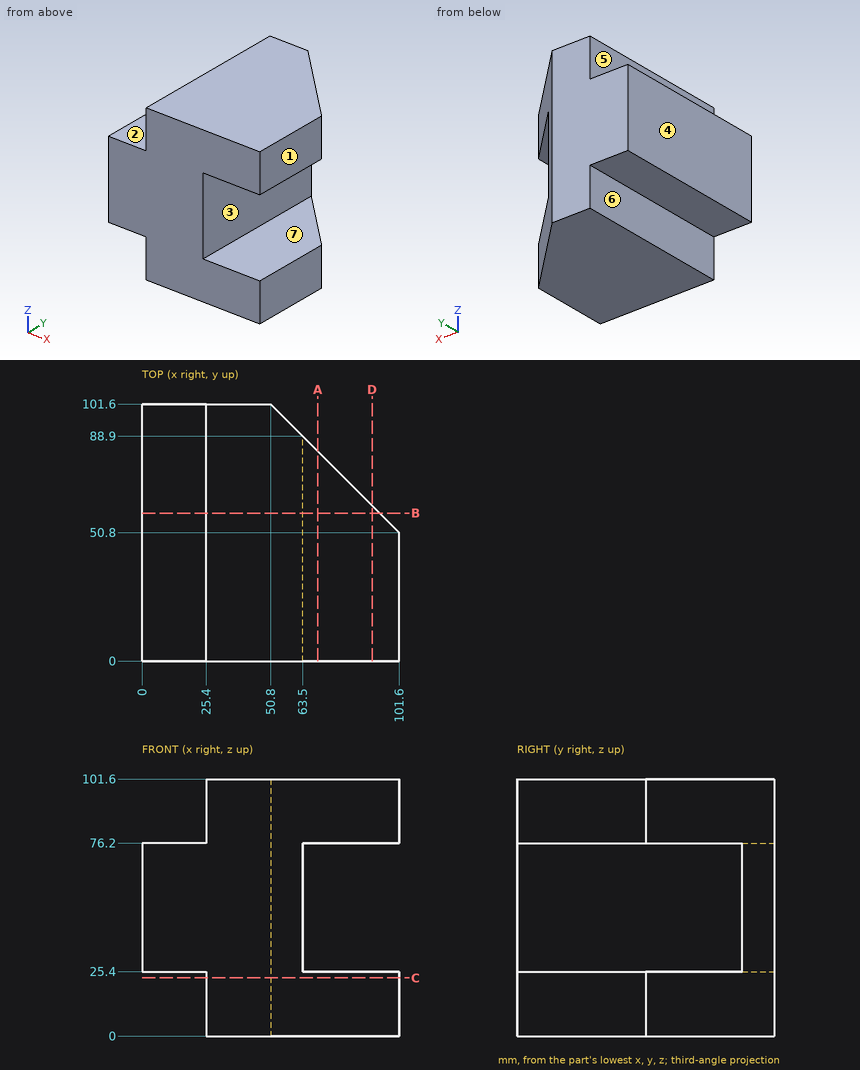
Part print with two shaded views. Sizes in mm from the minimum x, y, z corner. A direction names the side the tool comes from. Round coordinates to 2 decimals unless told otherwise and drop trailing zeros. Order: outer loops, then holes, each group sorted by start corner. A loop starts at its lowest first (then second) coordinate and runs counter-clockwise, first axis right, second up. Notation, with made-up numbers: M 13,66.5 L 24,66.5 A19 ccw 24,88.5 Z; hole C -3.75,-24.75 d7. An arc over 180 degrees is marked long. Use CSV: the item, a comma, the result in double quotes. Start each with the question number.
(1) Cut at B-B on y = 58.5. List the corners of the cut face in (x, z), then the cut area to 3 significant figures.
(2) Cut at D-D on x = 91. List the corners of the cut face in (y, z).
(3) Flat gauge pins, fed straight in: P1, Ø2, axis at x = 65, z = 67, coming from the -Y side (1 decimal); P2, Ø12.5, axis at x = 12, y = 64.5, coming from the +Z side; P3, Ø1, axis at y = 66.5, z = 79.5, coming from the +X side; P4, Ø15, axis at y = 36.5, z = 50, coming from the +X side. Where does each tip first touch, or does it go through?
(4) Cut at A-A on x = 69.5. List the corners of the cut face in (y, z), then the cut area to 3 significant figures.
(5) Mould opens along Z. For the marked faces 1, 2 and 3 say: +Z half, -Z half, draft (parallel to the pull), parting line (faces both ways), or undercut.
(6) Tool access for the marked faces 4, 5, 6 and 7: list every direction of +Z, -Z, +X, -X, +Y, -Y with a clear straight run to the whole face (end or side of a thin tool).
(7) Drill centre lines: probe 1 along Z at (x, y) = (96, 26); probe 2 along X at (y, z) = (61, 44.5); probe 3 along X at (y, z) = (25, 79). Where is each one in solid material? Low to high.
(8) Cut at C-C on z = 23. List the corners of the cut face in (x, y), then the cut area to 3 significant figures.
Findings:
1,outline,"M 0,25.4 L 25.4,25.4 L 25.4,0 L 93.9,0 L 93.9,25.4 L 63.5,25.4 L 63.5,76.2 L 93.9,76.2 L 93.9,101.6 L 25.4,101.6 L 25.4,76.2 L 0,76.2 Z"
1,area,"6,710 mm^2"
2,outline,"M 0,0 L 61.4,0 L 61.4,25.4 L 0,25.4 Z; M 0,76.2 L 61.4,76.2 L 61.4,101.6 L 0,101.6 Z"
3,P1,"passes through"
3,P2,"stops at z = 76.2"
3,P3,"stops at x = 86.4"
3,P4,"stops at x = 63.5"
4,outline,"M 0,0 L 82.9,0 L 82.9,25.4 L 0,25.4 Z; M 0,76.2 L 82.9,76.2 L 82.9,101.6 L 0,101.6 Z"
4,area,"4,210 mm^2"
5,face 1,"draft"
5,face 2,"+Z half"
5,face 3,"undercut"
6,face 4,"+Z, -Z, -X, +Y, -Y"
6,face 5,"+Z, -X, +Y, -Y"
6,face 6,"-Z, -X, +Y, -Y"
6,face 7,"+X, +Y, -Y"
7,probe 1,"z = 0 to 25.4, 76.2 to 101.6"
7,probe 2,"x = 0 to 63.5"
7,probe 3,"x = 25.4 to 101.6"
8,outline,"M 25.4,0 L 101.6,0 L 101.6,50.8 L 50.8,101.6 L 25.4,101.6 Z"
8,area,"6,450 mm^2"
